```python
from build123d import *

# Parameters (mm, degrees)
SKETCH1_W           = 128
SKETCH1_H           = 256
BOSS_EXTRUDE1_DEPTH = 13.56
BOSS_EXTRUDE1_DRAFT = -2
CUT_EXTRUDE1_DEPTH  = 10.84
SKETCH3_R           = 1.32
CUT_EXTRUDE2_DEPTH  = 10
FILLET1_R           = 10
FILLET2_R           = 2
CUT_EXTRUDE3_DEPTH  = 0.1


with BuildPart() as part:
    # Sketch1 → Boss-Extrude1 (with draft: the straight prism first)
    with BuildSketch(Plane.XY):
        Rectangle(SKETCH1_W, SKETCH1_H)
    extrude(amount=-BOSS_EXTRUDE1_DEPTH)
    # Boss-Extrude1: the draft: its side faces are tilted about the plane it starts from
    boss_extrude1_sides = [part.faces().sort_by_distance(p)[0] for p in [
        (0, -128, -6.78),
        (64, 0, -6.78),
        (0, 128, -6.78),
        (-64, 0, -6.78),
    ]]
    draft(boss_extrude1_sides, Plane.XY, BOSS_EXTRUDE1_DRAFT)

    # Sketch2 → Cut-Extrude1 (cut)
    with BuildSketch(Plane(origin=(0, 0, -13.56), x_dir=(-1, 0, 0), z_dir=(0, 0, -1))):
        Polygon((-52.526474366, -6.13), (52.526474366, -6.13), (52.526474366, -116.526474366), (17, -116.526474366), (17, -120.656474366), (-17, -120.656474366), (-17, -116.526474366), (-52.526474366, -116.526474366), align=None)
        Polygon((-52.526474366, 6.13), (-52.526474366, 116.526474366), (-17, 116.526474366), (-17, 120.656474366), (17, 120.656474366), (17, 116.526474366), (52.526474366, 116.526474366), (52.526474366, 6.13), align=None)
    extrude(amount=-CUT_EXTRUDE1_DEPTH, mode=Mode.SUBTRACT)

    # Sketch3 → Cut-Extrude2 (cut)
    with BuildSketch(Plane(origin=(0, 0, -13.56), x_dir=(-1, 0, 0), z_dir=(0, 0, -1))):
        with Locations((56, -120.026474366)):
            Circle(SKETCH3_R)
        with Locations((56, 0)):
            Circle(SKETCH3_R)
        with Locations(Location((56, 120.026474366, 0), (0, 0, 180))):
            Circle(SKETCH3_R)
        with Locations(Location((-56, -120.026474366, 0), (0, 0, 180))):
            Circle(SKETCH3_R)
        with Locations(Location((-56, 0, 0), (0, 0, 180))):
            Circle(SKETCH3_R)
        with Locations((-56, 120.026474366)):
            Circle(SKETCH3_R)
    extrude(amount=-CUT_EXTRUDE2_DEPTH, mode=Mode.SUBTRACT)

    # Fillet1
    fillet1_edges = [part.edges().sort_by_distance(p)[0] for p in [
        (52.526474366, 116.526474366, -8.14),
        (-52.526474366, 116.526474366, -8.14),
        (-52.526474366, -116.526474366, -8.14),
        (52.526474366, -116.526474366, -8.14),
    ]]
    fillet(fillet1_edges, radius=FILLET1_R)

    # Fillet2
    fillet2_edges = [part.edges().sort_by_distance(p)[0] for p in [
        (17, 116.526474366, -8.14),
        (17, 120.656474366, -8.14),
        (-17, 120.656474366, -8.14),
        (-17, 116.526474366, -8.14),
        (-17, -116.526474366, -8.14),
        (-17, -120.656474366, -8.14),
        (17, -120.656474366, -8.14),
        (17, -116.526474366, -8.14),
    ]]
    fillet(fillet2_edges, radius=FILLET2_R)

    # Sketch5 → Cut-Extrude3 (cut)
    with BuildSketch(Plane.XY):
        with BuildLine():
            ThreePointArc((0, 6.005906984), (41.00801644, 22.99198356), (57.994093016, 64))
            ThreePointArc((57.994093016, 64), (41.00801644, 105.00801644), (0, 121.994093016))
            ThreePointArc((0, 121.994093016), (18.969220237, 95.711668256), (25.674983731, 64))
            ThreePointArc((25.674983731, 64), (18.969220237, 32.288331744), (0, 6.005906984))
        make_face()
    extrude(amount=-CUT_EXTRUDE3_DEPTH, mode=Mode.SUBTRACT)


solid = part.part
```
Can you work these out from the model? Positions are in its coordinate system, mm. Round coordinates to 2 decimals unless told otherwise and drop trailing zeros. Loops run counter-clockwise (first coordinate to the right, second up) from the corner with the lowest first, then second, coordinate; pieces in that order, holes last.
Item 1: If we mould it in two halves opening along Y, with no side actions, what happens to faces 1 (the flat face through (4, 1, -13.56)), 2 (the flat face through (0, 120.656, -8))? For each: +Y half, -Y half, draft (parallel to the pull), parting line (faces both ways), or undercut.
Item 2: Suppose I cut it at A-A, the plane y = -49. Write out the boundary of the cut face in (x, z).
Item 3: Suppose I cut it at B-B, the plane x = -21.5. Write out the boundary of the cut face in (y, z).
Item 4: Suppose I cut it at C-C, the plane z = -6.75. State how many separate pieces and enclosed holes the cut face has, then the cut area to 3 significant figures.
Item 5: Will these pins go through, and if not, where does the flat tip stop? pin 1 Ø2 at (x, z) = (3.5, -4) entering from +Y; pin 2 Ø3.5 at (y, z) = (-56, -6) entering from +X; pin 3 Ø3 at (x, y) = (-56, -120.03) entering from +Z; pin 4 Ø1.5 at (x, z) = (-13, -12) entering from -Y.
Item 6: Suppose I cut it at D-D, the plane y = 80. Write out the boundary of the cut face in (x, z).
Item 7: Please list where these lines run through material, in increasing order: L1, parallel to Y at x = -56, z = -7; L2, parallel to Y at x = -47, z = -5.25; L3, parallel to Y at x = -57, z = -8.
Reported:
1. face 1: draft
1. face 2: undercut
2. outline: (-64, 0) - (-63.53, -13.56) - (-52.53, -13.56) - (-52.53, -2.72) - (52.53, -2.72) - (52.53, -13.56) - (63.53, -13.56) - (64, 0) - close
3. outline: (-128, 0) - (-127.53, -13.56) - (-116.53, -13.56) - (-116.53, -2.72) - (-6.13, -2.72) - (-6.13, -13.56) - (6.13, -13.56) - (6.13, -2.72) - (116.53, -2.72) - (116.53, -13.56) - (127.53, -13.56) - (128, 0) - close
4. separate pieces: 1
4. enclosed holes: 8
4. area: 9,160 mm2
5. pin 1: stops at y = 127.9
5. pin 2: stops at x = 63.85
5. pin 3: stops at z = 0
5. pin 4: stops at y = -127.61
6. outline: (-64, 0) - (-63.53, -13.56) - (-52.53, -13.56) - (-52.53, -2.72) - (52.53, -2.72) - (52.53, -13.56) - (63.53, -13.56) - (64, 0) - (55.74, 0) - (55.74, -0.1) - (24.02, -0.1) - (24.02, 0) - close
7. L1: y = -127.76 to -121.35, -118.71 to -1.32, 1.32 to 118.71, 121.35 to 127.76
7. L2: y = -127.82 to -115.47, -6.13 to 6.13, 115.47 to 127.82
7. L3: y = -127.72 to -120.89, -119.16 to -0.86, 0.86 to 119.16, 120.89 to 127.72
